Could you check a few things on this model? Use its own coordinates, in mm. Face numbers are marked on the shaded views. A direction names the side the tool comes from. Give positions to 0.01 mm unless a question says otherwise; leave off trailing zeros. Write each loop counter-clockwise with the first axis right and the second up, starting at its lowest first coordinate (ties: lowest second). Pieces come first, ordered by that corner, then holes. Notation, with made-up numbers: (33, 46.5) - (82, 46.5) arc R16 cw to (82, 51.5) - close; hole circle Ø10 at (79, -11.75). An arc over 180 degrees is marked (long way). Use one line per item in the form item = value.
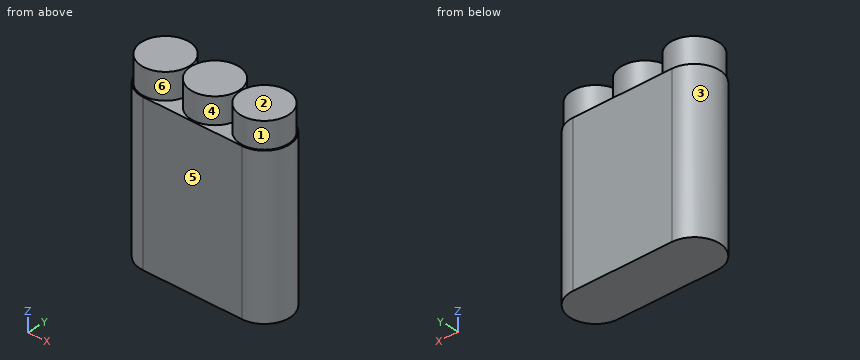
```python
from build123d import *

# Parameters (mm, degrees)
SKIZZE1_R                         = 9.25
AUFSATZ_LINEAR_AUSTRAGEN1_DEPTH   = 10
AUFSATZ_LINEAR_AUSTRAGEN1_2_DEPTH = 10
AUFSATZ_LINEAR_AUSTRAGEN1_3_DEPTH = 10
SKIZZE1_5_R                       = 9.25
AUFSATZ_LINEAR_AUSTRAGEN7_DEPTH   = 60


with BuildPart() as part:
    # Skizze1 → Aufsatz-Linear austragen1 (new body)
    with BuildSketch(Plane.XY):
        with Locations((-19, 0)):
            Circle(SKIZZE1_R)
    extrude(amount=AUFSATZ_LINEAR_AUSTRAGEN1_DEPTH)



with BuildPart() as body_2:
    # Skizze1 → Aufsatz-Linear austragen1 2 (new body)
    with BuildSketch(Plane.XY):
        Circle(SKIZZE1_R)
    extrude(amount=AUFSATZ_LINEAR_AUSTRAGEN1_2_DEPTH)


with BuildPart() as body_3:
    # Skizze1 → Aufsatz-Linear austragen1 3 (new body)
    with BuildSketch(Plane.XY):
        with Locations((19, 0)):
            Circle(SKIZZE1_R)
    extrude(amount=AUFSATZ_LINEAR_AUSTRAGEN1_3_DEPTH)


with BuildPart() as part_1:
    add(part.part)

    add(body_2.part)  # Aufsatz-Linear austragen7 merges body 2

    add(body_3.part)  # Aufsatz-Linear austragen7 merges body 3
    # Skizze1_5 → Aufsatz-Linear austragen7 (add)
    with BuildSketch(Plane.XY):
        with BuildLine():
            Line((-19, -9.75), (19, -9.75))
            ThreePointArc((19, -9.75), (28.75, 0), (19, 9.75))
            Line((19, 9.75), (-19, 9.75))
            ThreePointArc((-19, 9.75), (-28.75, 0), (-19, -9.75))
        make_face()
        Circle(SKIZZE1_5_R, mode=Mode.SUBTRACT)
        with Locations((19, 0)):
            Circle(SKIZZE1_5_R, mode=Mode.SUBTRACT)
        with Locations((-19, 0)):
            Circle(SKIZZE1_5_R, mode=Mode.SUBTRACT)
        with Locations((19, 0)):
            Circle(SKIZZE1_5_R)
        Circle(SKIZZE1_5_R)
        with Locations((-19, 0)):
            Circle(SKIZZE1_5_R)
    extrude(amount=-AUFSATZ_LINEAR_AUSTRAGEN7_DEPTH)


solid = part_1.part
```
1. Imagine slicing it at B-B, the plane y = -8. List the corners of the cut face in (x, z) for me.
Response values:
outline = (-24.57, -60) - (24.57, -60) - (24.57, 0) - (23.64, 0) - (23.64, 10) - (14.36, 10) - (14.36, 0) - (4.64, 0) - (4.64, 10) - (-4.64, 10) - (-4.64, 0) - (-14.36, 0) - (-14.36, 10) - (-23.64, 10) - (-23.64, 0) - (-24.57, 0) - close
2. If we mould it in two halves opening along X, with no side actions, what happens to the marked faces 3, 4, 5 and 6? For each: pulls with the +X half, pulls with the -X half, needs draft (parallel to the pull), parting line crosses it, or undercut.
Response values:
face_3 = pulls with the -X half
face_4 = undercut
face_5 = needs draft
face_6 = undercut
3. Which directions (+Z, -Z, +X, -X, +Y, -Y) give clear straight access to the entire face, cutting with the end or side of a thin tool? Please do the marked faces 1 and 2.
Response values:
face_1 = +Z
face_2 = +Z, +X, -X, +Y, -Y
4. Imagine slicing it at C-C, the plane z = -15.5. List the corners of the cut face in (x, y) for me.
Response values:
outline = (-19, -9.75) - (19, -9.75) arc R9.75 ccw to (19, 9.75) - (-19, 9.75) arc R9.75 ccw to start
5. Imagine slicing it at D-D, the plane y = 5.5. List the corners of the cut face in (x, z) for me.
Response values:
outline = (-27.05, -60) - (27.05, -60) - (27.05, 0) - (26.44, 0) - (26.44, 10) - (11.56, 10) - (11.56, 0) - (7.44, 0) - (7.44, 10) - (-7.44, 10) - (-7.44, 0) - (-11.56, 0) - (-11.56, 10) - (-26.44, 10) - (-26.44, 0) - (-27.05, 0) - close
6. If I drill on line 1 (Z direction, x = -9.5, y = 0.5); line 2 (X direction, y = 0, z = -43.5); line 3 (Y direction, x = -22.5, z = -42), over which ranges is the centre line in solid material (lowest first)? Write a range as from..to.
Response values:
line_1 = -60..0
line_2 = -28.75..28.75
line_3 = -9.1..9.1
7. Imagine slicing it at A-A, the plane x = 15. List the corners of the cut face in (y, z) for me, and give its area (3 significant figures).
Response values:
outline = (-9.75, -60) - (9.75, -60) - (9.75, 0) - (8.34, 0) - (8.34, 10) - (-8.34, 10) - (-8.34, 0) - (-9.75, 0) - close
area = 1,340 mm²
8. For pin 1 (4 mm diameter, centred on y = 3.5, z = -47, fed in from +X); pin 2 (3 mm diameter, centred on y = -3.5, z = -16, fed in from +X); pin 3 (1.5 mm diameter, centred on y = -4.5, z = -38, fed in from -X), each with a flat end and sliding along its axis, tell me the tip position at first contact or that it passes through.
Response values:
pin_1 = 28.63
pin_2 = 28.54
pin_3 = -28
